Verification items for the finished model (mm, model axes). A direction names the side the tool comes from. Coordinates: 2 decimals unless noted, no trailing zeros. Order: outer loops, then holes, each group sorted by start corner. A loop starts at its lowest first (then second) coordinate and runs counter-clockwise, first axis right, second up. Notation, with made-up numbers: (19, 7.25) -> (45, 7.25) arc R7 cw to (45, 12.25) -> close; hole circle Ø1 at (-15.5, 74). An arc over 180 degrees is marked (long way). Use CSV: the item, a comma, the result in double quotes. Start each with the question number.
1) Tool access check on faces 4 (the flat face through (128, 50, -12)), 5 (the flat face through (117, 120, 68)), 6 (the flat face through (26, -175, -12)). Record the directions out of +Z, -Z, +X, -X, +Y, -Y that give a thin tool (end or side, any length) a straight path to the whole face; none if there is none.
2) Scan lines: line 1 along Z through (x, y) = (-110, 2); line 2 along Y through (x, z) = (150, 18); line 3 along Y through (x, z) = (150, -17). Record each from-to range of solid material in increasing order.
3) Sectioned sample at C-C on z = 60.5. Record the boundary of the cut face in (x, y).
4) Release check for a two-part mould opening along Z. For faces 1 (the flat face through (-25, 137, 173)), 2 (the flat face through (-3, 3, -50)), 3 (the cylindrical face through (89.574, 47.87, -12.675)) record: released by +Z, released by -Z, zero draft, split by the parting line, or undercut.
5) Sectioned sample at A-A on x = 150. Record the boundary of the cut face in (y, z).
6) Go/stop test with flat-tipped pins: pin 1 (6 mm diameter, centred on y = -87.5, z = 129, fed in from -X); pin 2 (1.5 mm diameter, centred on y = 41.5, z = 135, fed in from +X); pin 3 (12 mm diameter, centred on x = -22, y = -59.5, fed in from +Z). Record where each tip stops, or that it passes through.
7) Sectioned sample at D-D on y = -67. Record the boundary of the cut face in (x, z).
8) Sectioned sample at B-B on y = -150. Record the boundary of the cut face in (x, z).
Autodesk Fusion 360 part; units mm, degrees
sketch "Sketch1" plane through (0, 0, 0) normal (0, 0, 1) x (1, 0, 0)
  line L0 (200, 200) -> (-200, 200)
  line L1 (-200, 200) -> (-200, -200)
  line L2 (-200, -200) -> (200, -200)
  line L3 (200, -200) -> (200, 200)
  line L4 (200, 200) -> (-200, -200) construction
  line L5 (200, -200) -> (100, -200)
  line L6 (100, -200) -> (100, -100)
  line L7 (100, -100) -> (200, -100)
  line L8 (200, -100) -> (200, -200)
  line L9 (-120, -200) -> (-120, -36.8544)
  line L10 (36.8544, 120) -> (200, 120)
  line L11 (-100, -200) -> (-100, -56.1738)
  line L12 (56.1738, 100) -> (200, 100)
  line L13 (-200, 200) -> (-100, 100) construction
  line L14 (-23.2233, 23.2233) -> (200, -200) construction
  arc A0 (-120, -36.8544) -> (36.8544, 120) centre (-200, 200) ccw
  arc A1 (-100, -56.1738) -> (56.1738, 100) centre (-200, 200) ccw
  line L15 (175, 100) -> (175, -100)
  line L16 (100, -175) -> (-100, -175)
  line L17 (-50, -175) -> (-50, -88.3141)
  arc A2 (-50, -88.3141) -> (88.3141, 50) centre (-200, 200) ccw
  line L18 (88.3141, 50) -> (175, 50)
  circle A3 centre (150, -150) radius 25
  circle A4 centre (150, -150) radius 15
  dimension "d1" = 400
  dimension "d2" = 400
  dimension "d3" = 100
  dimension "d4" = 100
  dimension "d5" = 500
  dimension "d6" = 550
  dimension "d7" = 80
  dimension "d8" = 80
  dimension "d10" = 25
  dimension "d11" = 25
  dimension "d13" = 50
  dimension "d14" = 30
  dimension "d15" = 50
extrude "Extrude1" add sketch "Sketch1" against normal blind 50 contours L0 L1 L2 L3 L9 L10 A0 | L2 L3 L9 L10 L11 L12 A0 A1 | L3 L7 L12 L15 | L2 L3 L5 L6 L7 L8 | L11 L12 A1 L15 L16 L17 A2 L18 | L2 L6 L11 L16 | L6 L7 L15 L16 L17 A2 L18 | A3 | A4
extrude "Extrude2" cut sketch "Sketch1" against normal blind 25 contours L6 L7 L15 L16 L17 A2 L18
extrude "Extrude3" cut sketch "Sketch1" against normal blind 110 contours A4
extrude "Extrude4" add sketch "Sketch1" along normal blind 25 contours L2 L3 L5 L6 L7 L8
extrude "Extrude5" add sketch "Sketch1" along normal blind 200 contours L2 L3 L9 L10 L11 L12 A0 A1
fillet "Fillet1" radius 25 4 edges at (-200, 200, -25) (200, 200, -25) (-200, -200, -25) (200, -200, -12.5)
fillet "Fillet2" radius 15 5 edges at (88.3141, 50, -12.5) (-50, -88.3141, -12.5) (-50, -175, -12.5) (100, -175, -12.5) (175, 50, -12.5)
sketch "Sketch2" plane through (0, -200, 0) normal (0, -1, 0) x (1, 0, 0)
  line L0 (175, -50) -> (175, 25)
  line L1 (175, 25) -> (100, 25)
  line L2 (100, 25) -> (100, 0)
  line L3 (100, 0) -> (-100, 0)
  line L4 (-100, 0) -> (-100, 200)
  line L5 (-100, 200) -> (-120, 200)
  line L6 (-120, 200) -> (-120, 0)
  line L7 (-120, 0) -> (-175, 0)
  line L8 (-175, 0) -> (-175, -50)
  line L9 (-175, -50) -> (175, -50)
  circle A0 centre (-110, 200) radius 62.5
  dimension "d30" = 125
extrude "Extrude6" add sketch "Sketch2" against normal blind 225 contours L4 L5 L6 A0 | L4 L5 L6 A0
sketch "Sketch3" plane through (200, 0, 0) normal (1, 0, 0) x (0, 1, 0)
  line L0 (-175, 25) -> (-175, -50)
  line L1 (-175, -50) -> (175, -50)
  line L2 (175, -50) -> (175, 0)
  line L3 (175, 0) -> (120, 0)
  line L4 (120, 0) -> (120, 200)
  line L5 (120, 200) -> (100, 200)
  line L6 (100, 200) -> (100, 0)
  line L7 (100, 0) -> (-100, 0)
  line L8 (-100, 0) -> (-100, 25)
  line L9 (-100, 25) -> (-175, 25)
  circle A0 centre (110, 200) radius 62.5
  dimension "d33" = 125
extrude "Extrude7" add sketch "Sketch3" against normal blind 225 contours L4 L5 L6 A0 | L4 L5 L6 A0
hole "Hole1" at (-110, -200, 200) direction (0, 1, 0) diameter 75 end through all
hole "Hole2" at (200, 110, 200) direction (-1, 0, 0) diameter 75 end through all
Answers follow:
1,face 4,"none"
1,face 5,"+X, -X, +Y"
1,face 6,"+Z"
2,line 1,"z = -50 to 0, 137.5 to 162.5, 237.5 to 262.5"
2,line 2,"y = -200 to -175, -125 to -100, 100 to 120"
2,line 3,"y = -200 to -165, -135 to -100, 50 to 200"
3,outline,"(-120, -200) -> (-100, -200) -> (-100, -56.17) arc R275 ccw to (56.17, 100) -> (200, 100) -> (200, 120) -> (36.85, 120) arc R250 cw to (-120, -36.85) -> close"
4,face 1,"zero draft"
4,face 2,"released by -Z"
4,face 3,"undercut"
5,outline,"(-200, -50) -> (-165, -50) -> (-165, 0) -> (-175, 0) -> (-175, 25) -> (-200, 25) -> close; (-135, -50) -> (200, -50) -> (200, 0) -> (120, 0) -> (120, 138.31) arc R62.5 ccw (long way) to (100, 138.31) -> (100, 0) -> (50, 0) -> (50, -25) -> (-100, -25) -> (-100, 25) -> (-125, 25) -> (-125, 0) -> (-135, 0) -> close; hole circle Ø75 at (110, 200)"
6,pin 1,"stops at x = -120"
6,pin 2,"stops at x = 25.26"
6,pin 3,"stops at z = 0"
7,outline,"(-200, -50) -> (200, -50) -> (200, 0) -> (175, 0) -> (175, -25) -> (-14.7, -25) -> (-14.7, 0) -> (-100, 0) -> (-100, 138.31) arc R62.5 ccw (long way) to (-120, 138.31) -> (-120, 0) -> (-200, 0) -> close; hole circle Ø75 at (-110, 200)"
8,outline,"(-200, -50) -> (135, -50) -> (135, 0) -> (125, 0) -> (125, 25) -> (100, 25) -> (100, -25) -> (-50, -25) -> (-50, 0) -> (-100, 0) -> (-100, 138.31) arc R62.5 ccw (long way) to (-120, 138.31) -> (-120, 0) -> (-200, 0) -> close; (165, -50) -> (200, -50) -> (200, 25) -> (175, 25) -> (175, 0) -> (165, 0) -> close; hole circle Ø75 at (-110, 200)"
